from build123d import *

# Parameters (mm, degrees)
SKETCH1_W           = 558.8
SKETCH1_H           = 304.8
BOSS_EXTRUDE1_DEPTH = 2.54
SKETCH2_W           = 558.8
SKETCH2_H           = 304.8
SKETCH2_W_2         = 553.72
SKETCH2_H_2         = 299.72
BOSS_EXTRUDE2_DEPTH = 19.05
FILLET1_R           = 2.54
SKETCH4_R           = 101.6
CUT_EXTRUDE2_DEPTH  = 19.05
BOSS_EXTRUDE3_START = 25.4
SKETCH5_R           = 107.95
SKETCH5_R_2         = 101.6
BOSS_EXTRUDE3_DEPTH = 25.4


with BuildPart() as part:
    # Sketch1 → Boss-Extrude1 (new body)
    with BuildSketch(Plane.XY):
        Rectangle(SKETCH1_W, SKETCH1_H)
    extrude(amount=BOSS_EXTRUDE1_DEPTH)

    # Sketch2 → Boss-Extrude2 (add)
    with BuildSketch(Plane.XY.offset(2.54)):
        Rectangle(SKETCH2_W, SKETCH2_H)
        Rectangle(SKETCH2_W_2, SKETCH2_H_2, mode=Mode.SUBTRACT)
    extrude(amount=-BOSS_EXTRUDE2_DEPTH)

    # Fillet1
    fillet1_edges = [part.edges().sort_by_distance(p)[0] for p in [
        (-279.4, 0, 2.54),
        (0, -152.4, 2.54),
        (279.4, 0, 2.54),
        (0, 152.4, 2.54),
    ]]
    fillet(fillet1_edges, radius=FILLET1_R)

    # Sketch4 → Cut-Extrude2 (cut)
    with BuildSketch(Plane.XY.offset(2.54)):
        Circle(SKETCH4_R)
    extrude(amount=-CUT_EXTRUDE2_DEPTH, mode=Mode.SUBTRACT)

    # Sketch5 → Boss-Extrude3 (add)
    with BuildSketch(Plane.XY.offset(2.54).offset(BOSS_EXTRUDE3_START)):
        with Locations(Location((0, 0, 0), (0, 0, 180))):
            Circle(SKETCH5_R)
        Circle(SKETCH5_R_2, mode=Mode.SUBTRACT)
    extrude(amount=-BOSS_EXTRUDE3_DEPTH)


solid = part.part
Can you work these out from the model? Positions are in its coordinate system, mm. A direction names the side the tool comes from. Give positions to 0.01 mm unless a question says otherwise; leave off trailing zeros. Loops run counter-clockwise (first coordinate to the right, second up) from the corner with the lowest first, then second, coordinate; pieces in that order, holes last. Notation, with made-up numbers: M 42,11.25 L 60,11.25 A19 ccw 60,45.25 Z; hole C -15.75,-10.75 d9. An arc over 180 degrees is marked long. One line per item, written item: value.
1) Imagine slicing it at A-A on y = 0. Write out the boundary of the cut face in (x, z).
Geometry check:
outline: M -279.4,-16.51 L -276.86,-16.51 L -276.86,0 L -101.6,0 L -101.6,27.94 L -107.95,27.94 L -107.95,2.54 L -276.86,2.54 A2.54 ccw -279.4,0 Z; M 101.6,0 L 276.86,0 L 276.86,-16.51 L 279.4,-16.51 L 279.4,0 A2.54 ccw 276.86,2.54 L 107.95,2.54 L 107.95,27.94 L 101.6,27.94 Z
2) Imagine slicing it at C-C on x = -130.5. Write out the boundary of the cut face in (y, z).
Geometry check:
outline: M -152.4,-16.51 L -149.86,-16.51 L -149.86,0 L 149.86,0 L 149.86,-16.51 L 152.4,-16.51 L 152.4,0 A2.54 ccw 149.86,2.54 L -149.86,2.54 A2.54 ccw -152.4,0 Z
3) On a 3-axis mill with a long thin cutter (end or side, diameter ignored), from which of +Z, -Z, +X, -X, +Y, -Y can I reach the whole of each face in a straight line? I mean faces 4 (the face through (-22.025, -99.184, 14.166)), 5 (the face through (-276.86, -2, -8)), 6 (the face through (79.56, -72.96, 15.42)). Say none if no direction works.
Geometry check:
face 4: +Z, -Z
face 5: -Z
face 6: +Z
4) Thinking about a two-plate mould opening in Y: for faces 1 (the face through (276.86, -2, -8)), 2 (the face through (-4, 152.4, -8)), 3 (the face through (279.4, -2, -8)), which applies, +Y half, -Y half, draft (parallel to the pull), parting line (faces both ways), or undercut?
Geometry check:
face 1: undercut
face 2: +Y half
face 3: draft
5) Please list where these lines run through material, in increasing order: line 1 (Y direction, x = 0, z = 19); line 2 (Y direction, x = 48, z = -9); line 3 (X direction, y = -128.5, z = -8).
Geometry check:
line 1: y = -107.95 to -101.6, 101.6 to 107.95
line 2: y = -152.4 to -149.86, 149.86 to 152.4
line 3: x = -279.4 to -276.86, 276.86 to 279.4
6) I'm going to push flat-ended pins straight in: pin 1 (2 mm diameter, centred on x = 51, z = 19.5, fed in from +Y); pin 2 (1 mm diameter, centred on y = -47, z = 18.5, fed in from +X); pin 3 (1.5 mm diameter, centred on y = -82, z = 19.5, fed in from -X). Where does each tip first touch, or does it pass through?
Geometry check:
pin 1: stops at y = 95.67
pin 2: stops at x = 97.42
pin 3: stops at x = -71.07
7) Imagine slicing it at D-D on y = -121. Write out the boundary of the cut face in (x, z), and give its area (3 significant figures).
Geometry check:
outline: M -279.4,-16.51 L -276.86,-16.51 L -276.86,0 L 276.86,0 L 276.86,-16.51 L 279.4,-16.51 L 279.4,0 A2.54 ccw 276.86,2.54 L -276.86,2.54 A2.54 ccw -279.4,0 Z
area: 1,500 mm²
8) Imagine slicing it at B-B on x = 0. Write out the boundary of the cut face in (y, z), and give its area (3 significant figures).
Geometry check:
outline: M -152.4,-16.51 L -149.86,-16.51 L -149.86,0 L -101.6,0 L -101.6,27.94 L -107.95,27.94 L -107.95,2.54 L -149.86,2.54 A2.54 ccw -152.4,0 Z; M 101.6,0 L 149.86,0 L 149.86,-16.51 L 152.4,-16.51 L 152.4,0 A2.54 ccw 149.86,2.54 L 107.95,2.54 L 107.95,27.94 L 101.6,27.94 Z
area: 662 mm²
